```python
from build123d import *

# Parameters (mm, degrees)
SKETCH1_W               = 203.2
SKETCH1_H               = 279.4
BOSS_EXTRUDE1_DEPTH     = 6.35
CUT_EXTRUDE1_START      = -7.35
SKETCH2_R               = 2.54
SKETCH2_W               = 25.4
SKETCH2_H               = 25.4
CUT_EXTRUDE1_DEPTH      = 8.35
MIRROR2_START           = -7.35
MIRROR2_COPY_1_SKETCH_R = 2.54
MIRROR2_COPY_1_SKETCH_W = 25.4
MIRROR2_COPY_1_SKETCH_H = 25.4
MIRROR2_COPY_1_DEPTH    = 8.35
SKETCH3_W               = 88.9
SKETCH3_H               = 44.45
CUT_EXTRUDE2_DEPTH      = 1
CUT_EXTRUDE2_DEPTH_BACK = 7.35


with BuildPart() as part:
    # Sketch1 → Boss-Extrude1 (new body)
    with BuildSketch(Plane(origin=(0, 0, 0), x_dir=(1, 0, 0), z_dir=(0, 1, 0))):
        Rectangle(SKETCH1_W, SKETCH1_H)
    extrude(amount=BOSS_EXTRUDE1_DEPTH)

    # Sketch2 → Cut-Extrude1 (cut)
    with BuildSketch(Plane(origin=(0, 6.35, 0), x_dir=(1, 0, 0), z_dir=(0, 1, 0)).offset(CUT_EXTRUDE1_START)):
        with Locations((-41.275, 55.88)):
            Circle(SKETCH2_R)
        with Locations((-41.275, 96.52)):
            Circle(SKETCH2_R)
        with Locations((-76.2, 55.88)):
            Circle(SKETCH2_R)
        with Locations((-96.52, 76.2)):
            Circle(SKETCH2_R)
        with Locations((-76.2, 96.52)):
            Circle(SKETCH2_R)
        with Locations((-76.2, 76.2)):
            Rectangle(SKETCH2_W, SKETCH2_H)
    cut_extrude1 = extrude(amount=CUT_EXTRUDE1_DEPTH, mode=Mode.SUBTRACT)

    # Mirror1: Cut-Extrude1 across plane
    add(cut_extrude1.mirror(Plane.XY), mode=Mode.SUBTRACT)

    # Mirror2: Cut-Extrude1 across plane
    add(cut_extrude1.mirror(Plane(origin=(0, 0, 0), x_dir=(0, 0, 1), z_dir=(1, 0, 0))), mode=Mode.SUBTRACT)

    # Mirror2 copy 1 sketch → Mirror2 copy 1 (cut)
    with BuildSketch(Plane(origin=(0, 6.35, 0), x_dir=(-1, 0, 0), z_dir=(0, 1, 0)).offset(MIRROR2_START)):
        with Locations((-41.275, 55.88)):
            Circle(MIRROR2_COPY_1_SKETCH_R)
        with Locations((-41.275, 96.52)):
            Circle(MIRROR2_COPY_1_SKETCH_R)
        with Locations((-76.2, 55.88)):
            Circle(MIRROR2_COPY_1_SKETCH_R)
        with Locations((-96.52, 76.2)):
            Circle(MIRROR2_COPY_1_SKETCH_R)
        with Locations((-76.2, 96.52)):
            Circle(MIRROR2_COPY_1_SKETCH_R)
        with Locations((-76.2, 76.2)):
            Rectangle(MIRROR2_COPY_1_SKETCH_W, MIRROR2_COPY_1_SKETCH_H)
    extrude(amount=MIRROR2_COPY_1_DEPTH, mode=Mode.SUBTRACT)

    # Sketch3 → Cut-Extrude2 (cut, two sides)
    with BuildSketch(Plane(origin=(32.763599602, 6.35, -4.611240895), x_dir=(0, 0, 1), z_dir=(0, 1, 0))) as cut_extrude2_sk:
        with Locations((-48.474759105, -32.763599602)):
            Rectangle(SKETCH3_W, SKETCH3_H)
        with Locations((97.321240895, -32.763599602)):
            Rectangle(SKETCH3_W, SKETCH3_H)
    extrude(amount=CUT_EXTRUDE2_DEPTH, mode=Mode.SUBTRACT)
    extrude(cut_extrude2_sk.sketch, amount=-CUT_EXTRUDE2_DEPTH_BACK, mode=Mode.SUBTRACT)


solid = part.part
```
Geometry check sheet. Reference: the model listing, model coordinates, mm. Round coordinates to 2 decimals unless told otherwise and drop trailing zeros. Write each loop counter-clockwise with the first axis right and the second up, starting at its lowest first coordinate (ties: lowest second). Pieces come first, ordered by that corner, then holes. Notation, with made-up numbers: (28.5, -34.5) -> (85.5, -34.5) arc R25 ccw to (85.5, -14.5) -> close; hole circle Ø2 at (24, 23.25). An arc over 180 degrees is marked (long way). Put each result on its own line as item: value.
1) Cross-section at B-B, the plane y = 3.5. Give the number of separate pieces and of enclosed holes in the cut face, plus the area to 3 significant figures.
Recorded:
separate pieces: 1
enclosed holes: 26
area: 45,900 mm2
2) Depth check by flat-ended pin: P1, Ø4, axis at x = 41.275, z = -55.88, coming from the -Y side. Enter the tip coordinate at first touch or a pass-through.
Recorded:
P1: passes through
3) Release check for a two-part mould opening along X. For faces 1 (the face through (-1, 0, -2)), 2 (the face through (-101.6, 3, 2)), 3 (the face through (22.225, 3, -54)) record: pulls with the +X half, pulls with the -X half, needs draft (parallel to the pull), parting line crosses it, or undercut.
Recorded:
face 1: needs draft
face 2: pulls with the -X half
face 3: undercut
4) Thickness scan on probe 1 along Z at (x, y) = (-96.52, 2.5); probe 2 along Z at (x, y) = (88, 4); probe 3 along X at (y, z) = (3, 80) (3 decimals). Record the ranges inside material, lowest first. Write a range as from..to.
Recorded:
probe 1: z = -139.7..-78.74, -73.66..73.66, 78.74..139.7
probe 2: z = -139.7..-88.9, -63.5..63.5, 88.9..139.7
probe 3: x = -101.6..-88.9, -63.5..-22.225, 22.225..63.5, 88.9..101.6
5) Cross-section at A-A, the plane z = 110. Enter the section's corners in (x, y) (3 decimals).
Recorded:
outline: (-101.6, 0) -> (-22.225, 0) -> (-22.225, 6.35) -> (-101.6, 6.35) -> close; (22.225, 0) -> (101.6, 0) -> (101.6, 6.35) -> (22.225, 6.35) -> close
